Geometry check sheet. Reference: the model listing, model coordinates, mm. Face numbers are marked on the shaded views. A direction names the side the tool comes from. Round coordinates to 2 decimals unless told otherwise and drop trailing zeros. Write each loop counter-clockwise with the first axis right and the second up, starting at its lowest first coordinate (ties: lowest second). Pieces come first, ordered by that corner, then holes. Notation, with made-up numbers: M 88.5,21.25 L 144.5,21.25 A18 cw 144.5,46.25 Z; hole C -10,-29 d8. An arc over 180 degrees is marked long. Put each result on its own line as item: value. Start each with the question number.
(1) Material ranges on probe 1 along Z at (x, y) = (48.45, 1.6) (3 decimals); probe 2 along X at (y, z) = (1.5, 8.5); probe 3 along Y at (x, z) = (32, 7), recorded low to high.
(2) Tool access check on the marked faces 4, 5, 6 and 7. Record the directions out of +Z, -Z, +X, -X, +Y, -Y that give a thin tool (end or side, any length) a straight path to the whole face; none if there is none.
(3) Section check A-A on z = 7.5. Record the cut outline in (x, y).
(4) Section check B-B on z = 30.15. Record the cut outline in (x, y) (3 decimals), then the cut area to 3 significant figures.
(5) Gauge pin test, flat ends, axial feed: pin 1 (3.5 mm diameter, centred on x = 45.5, y = 3, fed in from +Z); pin 2 (5.5 mm diameter, centred on y = -4.5, z = 35.5, fed in from +X); pin 3 (1.5 mm diameter, centred on y = 2, z = 23, fed in from -X); pin 4 (9 mm diameter, centred on x = 32.5, z = 20.5, fed in from -Y). Record the tip position at first contact, or that the pin passes through.
(6) Section check C-C on x = 43. Record the cut outline in (y, z), then the cut area to 3 significant figures.
(7) Section check D-D on y = 1.25. Record the cut outline in (x, z) (3 decimals).
(8) Mould release check, pull along Z, two halves, no side actions. Record for the marked faces 1, 2 and 3: pulls with the +Z half, pulls with the -Z half, needs draft (parallel to the pull), parting line crosses it, or undercut.
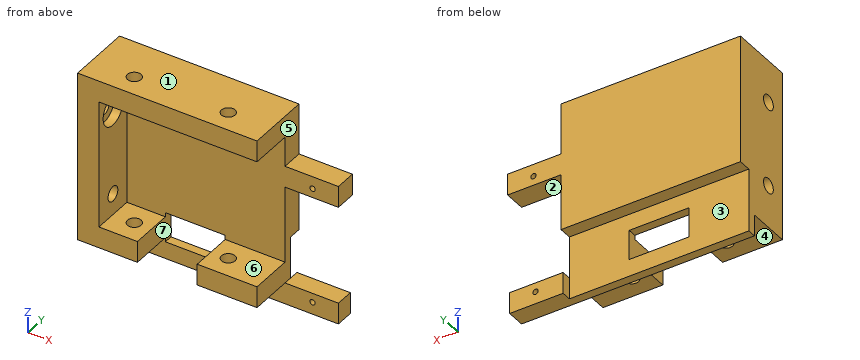
from build123d import *

# Parameters (mm, degrees)
SKETCH_1_W          = 42
SKETCH_1_H          = 45
EXTRUDE_1_DEPTH     = 5
SKETCH_2_W          = 42
SKETCH_2_H          = 5
EXTRUDE_2_DEPTH     = 10
SKETCH_3_R          = 1.6
CUT_EXTRUDE_1_DEPTH = 59.855755878
SKETCH_4_W          = 14
SKETCH_4_H          = 7
CUT_EXTRUDE_2_DEPTH = 64.356136246
SKETCH_5_W          = 42
SKETCH_5_H          = 14.838100381
CUT_EXTRUDE_3_DEPTH = 3
SKETCH_6_W          = 5
SKETCH_6_H          = 30
EXTRUDE_3_DEPTH     = 10
SKETCH_7_R          = 1.75
CUT_EXTRUDE_4_DEPTH = 60.110066825
SKETCH_8_R          = 3.5
CUT_EXTRUDE_5_DEPTH = 2
SKETCH_9_W          = 5
SKETCH_9_H          = 5
SKETCH_9_H_2        = 4.255093553
EXTRUDE_4_DEPTH     = 12.5
SKETCH_10_R         = 0.625
CUT_EXTRUDE_6_DEPTH = 72.381019886


with BuildPart() as part:
    # 草图1 → 凸台-拉伸1 (new body)
    with BuildSketch(Plane(origin=(0, 0, 0), x_dir=(1, 0, 0), z_dir=(0, 1, 0))):
        with Locations((21, -22.5)):
            Rectangle(SKETCH_1_W, SKETCH_1_H)
    extrude(amount=EXTRUDE_1_DEPTH)

    # 草图2 → 凸台-拉伸2 (add)
    with BuildSketch(Plane.XZ):
        with Locations((21, 42.5)):
            Rectangle(SKETCH_2_W, SKETCH_2_H)
        with Locations((21, 7.5)):
            Rectangle(SKETCH_2_W, SKETCH_2_H)
    extrude(amount=EXTRUDE_2_DEPTH)

    # 草图3 → 切除-拉伸1 (cut, through all)
    with BuildSketch(Plane(origin=(0, 0, 5), x_dir=(-1, 0, 0), z_dir=(0, 0, -1))):
        with Locations((-32, -5)):
            Circle(SKETCH_3_R)
        with Locations((-10, -5)):
            Circle(SKETCH_3_R)
    extrude(amount=-CUT_EXTRUDE_1_DEPTH, mode=Mode.SUBTRACT)

    # 草图4 → 切除-拉伸2 (cut, through all)
    with BuildSketch(Plane.XZ.offset(10)):
        with Locations((21, 7.5)):
            Rectangle(SKETCH_4_W, SKETCH_4_H)
    extrude(amount=-CUT_EXTRUDE_2_DEPTH, mode=Mode.SUBTRACT)

    # 草图5 → 切除-拉伸3 (cut)
    with BuildSketch(Plane(origin=(0, 5, 0), x_dir=(1, 0, 0), z_dir=(0, 1, 0))):
        with Locations((21, -7.419050191)):
            Rectangle(SKETCH_5_W, SKETCH_5_H)
    extrude(amount=-CUT_EXTRUDE_3_DEPTH, mode=Mode.SUBTRACT)

    # 草图6 → 凸台-拉伸3 (add)
    with BuildSketch(Plane.XZ):
        with Locations((2.5, 25)):
            Rectangle(SKETCH_6_W, SKETCH_6_H)
    extrude(amount=EXTRUDE_3_DEPTH)

    # 草图7 → 切除-拉伸4 (cut, through all)
    with BuildSketch(Plane(origin=(5, 0, 0), x_dir=(0, 0, -1), z_dir=(1, 0, 0))):
        with Locations((-35, -5)):
            Circle(SKETCH_7_R)
        with Locations((-15, -5)):
            Circle(SKETCH_7_R)
    extrude(amount=-CUT_EXTRUDE_4_DEPTH, mode=Mode.SUBTRACT)

    # 草图8 → 切除-拉伸5 (cut)
    with BuildSketch(Plane(origin=(5, 0, 0), x_dir=(0, 0, -1), z_dir=(1, 0, 0))):
        with Locations((-35, -5)):
            Circle(SKETCH_8_R)
    extrude(amount=-CUT_EXTRUDE_5_DEPTH, mode=Mode.SUBTRACT)

    # 草图9 → 凸台-拉伸4 (add)
    with BuildSketch(Plane(origin=(42, 0, 0), x_dir=(0, 0, -1), z_dir=(1, 0, 0))):
        with Locations((-30.5, 2.5)):
            Rectangle(SKETCH_9_W, SKETCH_9_H)
        with Locations((-2.5, 2.127546777)):
            Rectangle(SKETCH_9_W, SKETCH_9_H_2)
    extrude(amount=EXTRUDE_4_DEPTH)

    # 草图10 → 切除-拉伸6 (cut, through all)
    with BuildSketch(Plane.XZ):
        with Locations(Location((48.45, 30.15, 0), (0, 0, 270))):
            Circle(SKETCH_10_R)
        with Locations(Location((48.45, 2.85, 0), (0, 0, 270))):
            Circle(SKETCH_10_R)
    extrude(amount=-CUT_EXTRUDE_6_DEPTH, mode=Mode.SUBTRACT)


solid = part.part
Answers follow:
1. probe 1: z = 0 to 2.225, 3.475 to 5, 28 to 29.525, 30.775 to 33
1. probe 2: x = 0 to 14, 28 to 42
1. probe 3: y = -10 to -6.6, -3.4 to 2
2. face 4: -Z, +X, -X, -Y
2. face 5: +Z, +X, +Y, -Y
2. face 6: +X, -Y
2. face 7: +Y, -Y
3. outline: M 0,-10 L 14,-10 L 14,2 L 0,2 Z; M 28,-10 L 42,-10 L 42,2 L 28,2 Z; hole C 10,-5 d3.2; hole C 32,-5 d3.2
4. outline: M 0,-10 L 5,-10 L 5,0 L 47.825,0 L 47.825,5 L 0,5 Z; M 49.075,0 L 54.5,0 L 54.5,5 L 49.075,5 Z
4. area: 316 mm^2
5. pin 1: stops at z = 33
5. pin 2: stops at x = 3
5. pin 3: stops at x = 0
5. pin 4: stops at y = 0
6. outline: M 0,0 L 4.26,0 L 4.26,5 L 0,5 Z; M 0,28 L 5,28 L 5,33 L 0,33 Z
6. area: 46.3 mm^2
7. outline: M 0,0 L 54.5,0 L 54.5,5 L 42,5 L 42,28 L 54.5,28 L 54.5,33 L 42,33 L 42,45 L 0,45 Z; hole M 14,4 L 28,4 L 28,11 L 14,11 Z; hole C 48.45,2.85 d1.25; hole C 48.45,30.15 d1.25
8. face 1: pulls with the +Z half
8. face 2: undercut
8. face 3: needs draft
